Check sheet for the modelled part. Datum: model origin and axes. Units: mm. A direction names the side the tool comes from. Give positions to 0.01 mm unless a question says otherwise; leave off trailing zeros. Order: outer loops, then holes, each group sorted by start corner. A loop starts at its lowest first (then second) coordinate and runs counter-clockwise, first axis right, second up.
Autodesk Inventor part; units mm, degrees
ref_plane "YZ Plane" through (0, 0, 0) normal (1, 0, 0) x (0, 1, 0)
ref_plane "XZ Plane" through (0, 0, 0) normal (0, 1, 0) x (-1, 0, 0)
ref_plane "XY Plane" through (0, 0, 0) normal (0, 0, 1) x (1, 0, 0)
sketch "Sketch1" plane through (0, 0, 0) normal (1, 0, 0) x (0, 1, 0)
  line L0 (0, 0) -> (12, 0)
  line L1 (12, 0) -> (12, 10)
  line L2 (12, 10) -> (0, 10)
  line L3 (0, 10) -> (0, 0)
  line L4 (-105, -3) -> (15, -3)
  line L5 (15, -3) -> (15, 13)
  line L6 (15, 13) -> (-105, 13)
  line L7 (-105, 13) -> (-105, -3)
  point P0 (0, 5)
  dimension "d0" = 12
  dimension "d1" = 10
  dimension "d4" = 16
  dimension "d5" = 3
  dimension "d6" = 120
  dimension "d7" = 3
extrude "Extrusion1" add sketch "Sketch1" along normal blind 10
sketch "Sketch2" plane through (10, 0, 0) normal (1, 0, 0) x (0, 0, -1)
  circle A0 centre (-5, -92) radius 1.6
  circle A1 centre (-5, -55) radius 1.6
  line L0 (0, 0) -> (-10, 0)
  line L1 (3, -105) -> (3, 15)
  dimension "d14" = 3.2
  dimension "d15" = 3.2
  dimension "d16" = 55
  dimension "d17" = 37
  dimension "d18" = 8
  dimension "d19" = 8
extrude "Extrusion2" cut sketch "Sketch2" against normal blind 6
sketch "Sketch3" plane through (0, 0, 0) normal (-1, 0, 0) x (0, 0, 1)
  line L0 (10, 0) -> (0, 0) construction
  line L1 (8, -15) -> (11, -15)
  line L2 (11, -15) -> (11, -55)
  line L3 (11, -55) -> (8, -55)
  line L4 (8, -55) -> (8, -15)
  line L5 (13, 15) -> (13, -105)
  line L6 (-3, 15) -> (13, 15)
  dimension "d22" = 3
  dimension "d23" = 40
  dimension "d24" = 2
  dimension "d25" = 30
extrude "Extrusion4" add sketch "Sketch3" along normal blind 20
fillet "Fillet2" radius 6 2 edges at (-20, -55, 9.5) (-20, -15, 9.5)
sketch "Sketch4" plane through (0, -55, 11) normal (0, 0, 1) x (1, 0, 0)
  circle A0 centre (-10, 10) radius 1.6
  circle A1 centre (-10, 30) radius 1.6
  line L0 (0, 70) -> (0, -50)
  line L1 (0, 0) -> (-14, 0)
  line L2 (0, 40) -> (-14, 40)
  point P0 (0, 55)
  dimension "d35" = 3.2
  dimension "d36" = 3.2
  dimension "d37" = 10
  dimension "d38" = 10
  dimension "d39" = 10
  dimension "d40" = 10
fillet "Fillet3" radius 2 4 edges at (5, -105, 13) (5, 15, 13) (5, 15, -3) (5, -105, -3)
extrude "Extrusion5" cut sketch "Sketch4" against normal through all
equation "\"d5\" = -0.5 * d1 + 0.5 * d4"
equation "\"d7\" = d5"
equation "\"d19\" = d18"
equation "\"d38\" = d37"
equation "\"d40\" = d39"
properties part number "Wheel IR Holder LH"
1) Draft check along Z on faces 6 (the face through (7.042, -90.414, 5.208)), 7 (the face through (5.07, 14.43, 12.4)), 8 (the face through (-7, -55, 10)). Enter one of: +Z half, -Z half, draft (parallel to the pull), parting line (faces both ways), or undercut.
Recorded:
face 6: undercut
face 7: +Z half
face 8: draft
2) Section check D-D, the plane y = 4. Record the cut outline in (x, z).
Recorded:
outline: (0, -3) - (10, -3) - (10, 0) - (0, 0) - close; (0, 10) - (10, 10) - (10, 13) - (0, 13) - close
3) Material ranges on L1, parallel to Y at x = 8.35, z = 5; L2, parallel to Y at x = 3.25, z = 2.5; L3, parallel to Z at x = 0.5, y = 2, recorded low to high.
Recorded:
L1: y = -105 to -93.6, -90.4 to -56.6, -53.4 to 0, 12 to 15
L2: y = -105 to 0, 12 to 15
L3: z = -3 to 0, 10 to 13
4) Section check B-B, the plane z = 1. Record the cut outline in (x, y), then the cut area to 3 significant figures.
Recorded:
outline: (0, -105) - (10, -105) - (10, 0) - (0, 0) - close; (0, 12) - (10, 12) - (10, 15) - (0, 15) - close
area: 1,080 mm2
5) Section check A-A, the plane x = -10. Record the cut outline in (y, z).
Recorded:
outline: (-55, 8) - (-46.6, 8) - (-46.6, 11) - (-55, 11) - close; (-43.4, 8) - (-26.6, 8) - (-26.6, 11) - (-43.4, 11) - close; (-23.4, 8) - (-15, 8) - (-15, 11) - (-23.4, 11) - close
6) Depth check by flat-ended pin: pin 1 Ø1.9 at (x, y) = (-10, -25) entering from -Z; pin 2 Ø1 at (x, z) = (-11.5, 10) entering from -Y; pin 3 Ø5 at (y, z) = (-64, 1.5) entering from -X; pin 4 Ø3.5 at (x, y) = (-10, -45) entering from +Z. Enter the tip coordinate at first touch or a pass-through.
Recorded:
pin 1: passes through
pin 2: stops at y = -55
pin 3: stops at x = 0
pin 4: stops at z = 11
7) Set-up check for faces 1 (the face through (4, -55, 5)), 2 (the face through (5, 6, 10)), 3 (the face through (-10, -35, 11)), 4 (the face through (5.07, -104.4, 12.43)), 5 (the face through (-7, -15, 9)): record each of +Z, -Z, +X, -X, +Y, -Y from which the full face is reachable in a straight line by a thin tool's end or side.
Recorded:
face 1: +X
face 2: +X, -X
face 3: +Z, -X, +Y, -Y
face 4: +Z, +X, -X, -Y
face 5: +Z, -Z, -X, +Y
8) Section check C-C, the plane y = -45. Record the cut outline in (x, z), then the cut area to 3 significant figures.
Recorded:
outline: (-20, 8) - (-11.6, 8) - (-11.6, 11) - (-20, 11) - close; (-8.4, 8) - (0, 8) - (0, -3) - (10, -3) - (10, 13) - (0, 13) - (0, 11) - (-8.4, 11) - close
area: 210 mm2
